from build123d import *

# Parameters (mm, degrees)
BOSS_EXTRU_1_DEPTH = 0.5
BOSS_EXTRU_2_DEPTH = 1.5
BOSS_EXTRU_3_START = -55
BOSS_EXTRU_3_DEPTH = 1.5


with BuildPart() as part:
    # Esquisse1 → Boss.-Extru.1 (new body)
    with BuildSketch(Plane.XY):
        with BuildLine():
            Line((-28.25, 0), (28.25, 0))
            Line((28.25, 0), (28.25, -7))
            Line((28.25, -7), (26.75, -7))
            Line((26.75, -7), (26.75, -9))
            Line((26.75, -9), (28.25, -9))
            Line((28.25, -9), (28.25, -16))
            Line((28.25, -16), (26.75, -16))
            Line((26.75, -16), (26.75, -18))
            Line((26.75, -18), (28.25, -18))
            Line((28.25, -18), (28.25, -23.155433616))
            ThreePointArc((28.25, -23.155433616), (13.925220168, -27.365070972), (1.753926702, -18.717529168))
            ThreePointArc((1.753926702, -18.717529168), (0, -17.678643691), (-1.753926702, -18.717529168))
            ThreePointArc((-1.753926702, -18.717529168), (-13.925220168, -27.365070972), (-28.25, -23.155433616))
            Line((-28.25, -23.155433616), (-28.25, -18))
            Line((-28.25, -18), (-26.75, -18))
            Line((-26.75, -18), (-26.75, -16))
            Line((-26.75, -16), (-28.25, -16))
            Line((-28.25, -16), (-28.25, -9))
            Line((-28.25, -9), (-26.75, -9))
            Line((-26.75, -9), (-26.75, -7))
            Line((-26.75, -7), (-28.25, -7))
            Line((-28.25, -7), (-28.25, 0))
        make_face()
    extrude(amount=BOSS_EXTRU_1_DEPTH)

    # Esquisse2 → Révolution1 (revolve)
    with BuildSketch(Plane.XZ.offset(10.5), mode=Mode.PRIVATE) as r_volution1_sk:
        Polygon((-16.75, 0), (-16.75, 2.2), (-12.75, 2.2), (-10.25, 0), align=None)
    revolve(r_volution1_sk.sketch.rotate(Axis((-16.75, -10.5, 0), (0, 0, 1)), 180), axis=Axis((-16.75, -10.5, 0), (0, 0, 1)))

    # Esquisse3 → Révolution2 (revolve)
    with BuildSketch(Plane.XZ.offset(10.5), mode=Mode.PRIVATE) as r_volution2_sk:
        Polygon((16.75, 0), (16.75, 2.2), (20.75, 2.2), (23.25, 0), align=None)
    revolve(r_volution2_sk.sketch.rotate(Axis((16.75, -10.5, 0), (0, 0, 1)), 180), axis=Axis((16.75, -10.5, 0), (0, 0, 1)))

    # Esquisse5 → Boss.-Extru.2 (add)
    with BuildSketch(Plane(origin=(28.25, 0, 0), x_dir=(0, 0, -1), z_dir=(1, 0, 0))):
        Polygon((0, -18), (-1.119243945, -16), (-1.5, -16.213079455), (-0.5, -18), align=None)
        Polygon((-0.5, -9), (-1.5, -7.213079455), (-1.119243945, -7), (0, -9), align=None)
    extrude(amount=-BOSS_EXTRU_2_DEPTH)

    # Esquisse5<2> → Boss.-Extru.3 (add)
    with BuildSketch(Plane(origin=(28.25, 0, 0), x_dir=(0, 0, -1), z_dir=(1, 0, 0)).offset(BOSS_EXTRU_3_START)):
        Polygon((0, -18), (-1.119243945, -16), (-1.5, -16.213079455), (-0.5, -18), align=None)
        Polygon((-0.5, -9), (-1.5, -7.213079455), (-1.119243945, -7), (0, -9), align=None)
    extrude(amount=-BOSS_EXTRU_3_DEPTH)


solid = part.part
Can you work these out from the model? Positions are in its coordinate system, mm. A direction names the side the tool comes from. Round coordinates to 2 decimals unless told otherwise and drop trailing zeros. Loops run counter-clockwise (first coordinate to the right, second up) from the corner with the lowest first, then second, coordinate; pieces in that order, holes last. Notation, with made-up numbers: (51.25, -14) - (59.25, -14) arc R16 cw to (59.25, -3) - close; hole circle Ø11 at (-40, 70.25). An arc over 180 degrees is marked (long way). Answer in a Markdown table with one row per item. Add a question column.
Q1. I need wall thicknesses on L1, parallel to Z at x = 26, y = -5; L2, parallel to X at y = -9.25, z = 1.8; L3, parallel to X at y = -24.25, z = 0.2. Which ranges of each line are inside material? Lowest first, please.
Q2. I want a section at D-D on x = 9. List the corners of the cut face in (y, z) for me.
Q3. I want a section at C-C on y = -19.25. List the corners of the cut face in (x, z) for me.
Q4. I want a section at A-A on y = -10.5. List the corners of the cut face in (x, z) for me, and give its area (3 significant figures).
Q5. I want a section at B-B on x = 16.75. List the corners of the cut face in (y, z) for me, and give its area (3 significant figures).
Q6. For pin 1 Ø1.5 at (x, y) = (-10.5, -9) entering from +Z; pin 2 Ø0.6 at (y, z) = (-8, 0) entering from +X; pin 3 Ø0.6 at (x, z) = (-27.5, 0.5) entering from -Y, each with a flat end and sliding along its axis, tell me the tip position at first contact or that it passes through.
Q7. We'd pull the mould along X, two halves only. Please class faces 4 (the flat face through (28.25, -19.6, 0.2)), 5 (the flat face through (-28.25, -11.5, 0.2)), 6 (the cylindrical face through (14.14, -27.4, 0.25)), 7 (the flat face through (-27.49, -8.119, 0.993)): pulls with the +X half, pulls with the -X half, needs draft (parallel to the pull), parting line crosses it, or undercut.
Q8. Which directions (+Z, -Z, +X, -X, +Y, -Y) give clear straight access to the entire face, cutting with the end or side of a thin tool? Please do faces 1 (the cylindrical face through (0.03, -17.68, 0.25)), 2 (the flat face through (26.75, -7.8, 0.9)), 3 (the flat face through (27.51, -8.119, 0.993)).
A:
| question | item | result |
|---|---|---|
| 1 | L1 | 0 to 0.5 |
| 1 | L2 | -21.03 to -12.47, 12.47 to 21.03 |
| 1 | L3 | -26.92 to -6.58, 6.58 to 26.92 |
| 2 | outline | (-25.74, 0) - (0, 0) - (0, 0.5) - (-25.74, 0.5) - close |
| 3 | outline | (-28.25, 0) - (-2.06, 0) - (-2.06, 0.5) - (-28.25, 0.5) - close; (2.06, 0) - (28.25, 0) - (28.25, 0.5) - (2.06, 0.5) - close |
| 4 | outline | (-28.25, 0) - (28.25, 0) - (28.25, 0.5) - (22.68, 0.5) - (20.75, 2.2) - (12.75, 2.2) - (10.82, 0.5) - (-10.82, 0.5) - (-12.75, 2.2) - (-20.75, 2.2) - (-22.68, 0.5) - (-28.25, 0.5) - close |
| 4 | area | 62.0 mm^2 |
| 5 | outline | (-27.6, 0) - (0, 0) - (0, 0.5) - (-4.57, 0.5) - (-6.5, 2.2) - (-14.5, 2.2) - (-16.43, 0.5) - (-27.6, 0.5) - close |
| 5 | area | 30.7 mm^2 |
| 6 | pin 1 | z = 0.72 |
| 6 | pin 2 | x = 26.75 |
| 6 | pin 3 | y = -24.04 |
| 7 | face 4 | pulls with the +X half |
| 7 | face 5 | pulls with the -X half |
| 7 | face 6 | undercut |
| 7 | face 7 | needs draft |
| 8 | face 1 | +Z, -Z, -Y |
| 8 | face 2 | +Z, +Y, -Y |
| 8 | face 3 | +Z, +X |
